Model file for the job. Use its own axes, mm. Coordinates: 2 decimals unless noted, no trailing zeros. Order: outer loops, then holes, each group sorted by start corner. A loop starts at its lowest first (then second) coordinate and runs counter-clockwise, first axis right, second up. Notation, with made-up numbers: (47.5, 51.5) -> (84.5, 51.5) arc R16 ccw to (84.5, 82.5) -> close; hole circle Ø8 at (7.5, 87.5). An arc over 180 degrees is marked (long way). Return JSON: item names as keys, results as strings. Group by question number.
1) Cut at A-A (x = -222). Write the cut outline in (y, z).
2) Probe line 1 (X direction, y = 8.5, z = 57); line 2 (Z direction, x = 365, y = 2.5); line 3 (Z direction, x = -155, y = -1.25). List the from-to ranges inside material, lowest first.
3) Cut at B-B (z = 23). Write the cut outline in (x, y), and give its area (3 significant figures).
4) Cut at C-C (y = -0.75). Write the cut outline in (x, z), and give its area (3 significant figures).
5) Flat gauge pins, fed straight in: pin 1 (10 mm diameter, centred on y = -10.5, z = 139.5, fed in from +X); pin 2 (6 mm diameter, centred on y = 2.5, z = 67, fed in from +X); pin 3 (2 mm diameter, centred on y = -1.5, z = 73.5, fed in from +X). Where does each tip first touch, or does it go through?
from build123d import *

# Parameters (mm, degrees)
EXTRUDE1_DEPTH          = 490
CUT_EXTRUDE1_DEPTH      = 11
CUT_EXTRUDE1_DEPTH_BACK = 16
CUT_EXTRUDE2_DEPTH      = 11
CUT_EXTRUDE2_DEPTH_BACK = 16


with BuildPart() as part:
    # Sketch1 → Extrude1 (new body, symmetric)
    with BuildSketch(Plane(origin=(0, 0, 0), x_dir=(0, 0, -1), z_dir=(1, 0, 0))):
        Polygon((-200, -7), (-200, -15), (0, -15), (0, 10), (-157.923523492, 10), align=None)
    extrude(amount=EXTRUDE1_DEPTH, both=True)

    # Sketch2 → Cut-Extrude1 (cut, two sides)
    with BuildSketch(Plane(origin=(0, 0, 0), x_dir=(1, 0, 0), z_dir=(0, 1, 0))) as cut_extrude1_sk:
        Polygon((-335.776225586, 2005.502726748), (-476.014637611, 0), (-490, -200), (-630.238412025, -2205.502726748), (-4641.243865521, -1925.025902697), (-4346.781679081, 2285.979550799), align=None)
    extrude(amount=CUT_EXTRUDE1_DEPTH, mode=Mode.SUBTRACT)
    extrude(cut_extrude1_sk.sketch, amount=-CUT_EXTRUDE1_DEPTH_BACK, mode=Mode.SUBTRACT)

    # Sketch3 → Cut-Extrude2 (cut, two sides)
    with BuildSketch(Plane(origin=(0, 0, 0), x_dir=(1, 0, 0), z_dir=(0, 1, 0))) as cut_extrude2_sk:
        Polygon((630.238412025, -2205.502726748), (490, -200), (476.014637611, 0), (335.776225586, 2005.502726748), (4346.781679081, 2285.979550799), (4641.243865521, -1925.025902697), align=None)
    extrude(amount=CUT_EXTRUDE2_DEPTH, mode=Mode.SUBTRACT)
    extrude(cut_extrude2_sk.sketch, amount=-CUT_EXTRUDE2_DEPTH_BACK, mode=Mode.SUBTRACT)


solid = part.part
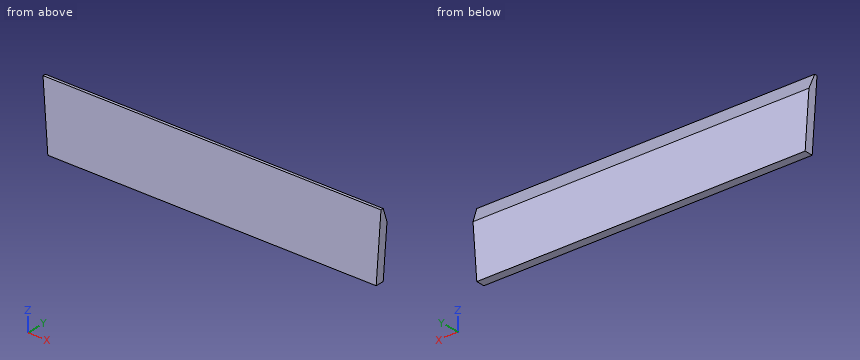
Answers below:
{
 "1": {"outline": "(-15, 0) -> (10, 0) -> (10, 157.92) -> (-7, 200) -> (-15, 200) -> close"},
 "2": {"line 1": "x = -480 to 480", "line 2": "z = 0 to 176.49", "line 3": "z = 0 to 185.77"},
 "3": {"outline": "(-477.62, -15) -> (477.62, -15) -> (477.62, 10) -> (-477.62, 10) -> close", "area": "23,900 mm^2"},
 "4": {"outline": "(-488.92, 184.53) -> (-476.01, 0) -> (476.01, 0) -> (488.92, 184.53) -> close", "area": "178,000 mm^2"},
 "5": {"pin 1": "stops at x = 486.12", "pin 2": "stops at x = 480.91", "pin 3": "stops at x = 481.22"}
}
